Can you work these out from the model? Positions are in its coordinate system, mm. Face numbers are marked on the shaded views. A direction names the side the tool comes from. Give positions to 0.01 mm unless a question says otherwise; leave off trailing zeros. Loops run counter-clockwise (first coordinate to the right, second up) from the corner with the lowest first, then second, coordinate; pieces in that order, holes last. Notation, with made-up numbers: (36.25, 16.25) - (94.25, 16.25) arc R36 cw to (94.25, 51.25) - close; hole circle Ø10 at (16.25, 34). An arc over 180 degrees is marked (long way). Write item = value, one per line.
from build123d import *

# Parameters (mm, degrees)
RESSALTO_EXTRUS_O1_DEPTH      = 0.8
RESSALTO_EXTRUS_O2_DEPTH      = 1
RESSALTO_EXTRUS_O2_DEPTH_BACK = 6


with BuildPart() as part:
    # Esboço1 → Ressalto-extrusão1 (new body)
    with BuildSketch(Plane.XY):
        Polygon((8.5, 13.5), (-8.5, 13.5), (-8.5, -13.5), (-6.5, -13.5), (-6.5, -11.5), (6.5, -11.5), (6.5, -13.5), (8.5, -13.5), align=None)
    extrude(amount=RESSALTO_EXTRUS_O1_DEPTH)

    # Esboço3 → Ressalto-extrusão2 (add, two sides)
    with BuildSketch(Plane(origin=(0, 13.5, 0), x_dir=(1, 0, 0), z_dir=(0, 1, 0))) as ressalto_extrus_o2_sk:
        with BuildLine():
            Line((-3, 3), (3, 3))
            ThreePointArc((3, 3), (4.5, 1.5), (3, 0))
            Line((3, 0), (-3, 0))
            ThreePointArc((-3, 0), (-4.5, 1.5), (-3, 3))
        make_face()
    extrude(amount=RESSALTO_EXTRUS_O2_DEPTH)
    extrude(ressalto_extrus_o2_sk.sketch, amount=-RESSALTO_EXTRUS_O2_DEPTH_BACK)


solid = part.part
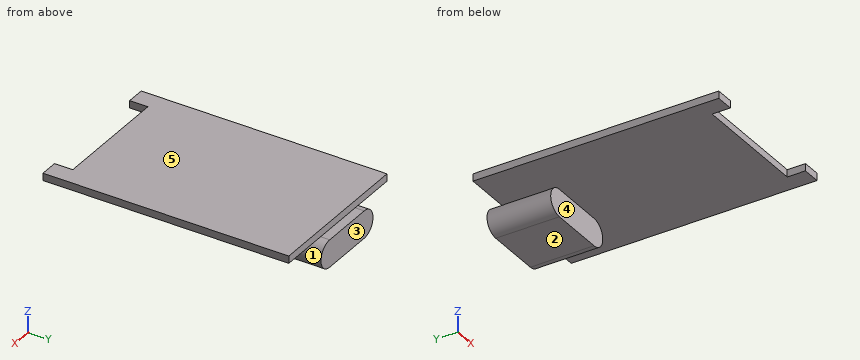
Q1. For pin 1 (8.5 mm diameter, centred on x = -1.5, y = -4.5, fed in from -Z); pin 2 (0.9 mm diameter, centred on x = 1.5, z = -1, fed in from -Y); pin 3 (0.8 mm diameter, centred on x = 1, y = 14, fed in from +Z), each with a flat end and sliding along its axis, tell me the tip position at first contact or that it passes through.
Output:
pin_1 = 0
pin_2 = 7.5
pin_3 = 0
Q2. Imagine slicing it at B-B, the plane y = -3.5. Write out the boundary of the cut face in (x, z), then the cut area to 3 significant figures.
Output:
outline = (-8.5, 0) - (8.5, 0) - (8.5, 0.8) - (-8.5, 0.8) - close
area = 13.6 mm2
Q3. Imagine slicing it at A-A, the plane z = 0.5. Write out the boundary of the cut face in (x, y), then the cut area to 3 significant figures.
Output:
outline = (-8.5, -13.5) - (-6.5, -13.5) - (-6.5, -11.5) - (6.5, -11.5) - (6.5, -13.5) - (8.5, -13.5) - (8.5, 13.5) - (-8.5, 13.5) - close
area = 433 mm2
Q4. We'd pull the mould along Z, two halves only. Please class the marked faces 1, 2 and 3: released by +Z, released by -Z, zero draft, split by the parting line, or undercut.
Output:
face_1 = undercut
face_2 = released by -Z
face_3 = zero draft
Q5. I need wall thicknesses on L1, parallel to Z at x = 6.25, y = -10.75; L2, parallel to Y at x = -2.25, z = -0.05; L3, parallel to Y at x = 0.25, z = 0.2. Which ranges of each line are inside material? Lowest first, please.
Output:
L1 = 0 to 0.8
L2 = 7.5 to 14.5
L3 = -11.5 to 13.5
Q6. Which directions (+Z, -Z, +X, -X, +Y, -Y) give clear straight access to the entire face, cutting with the end or side of a thin tool? Please do the marked faces 4 and 5.
Output:
face_4 = -Z, +X, -X, -Y
face_5 = +Z, +X, -X, +Y, -Y
Q7. Imagine slicing it at C-C, the plane x = 6. Write out the boundary of the cut face in (y, z).
Output:
outline = (-11.5, 0) - (13.5, 0) - (13.5, 0.8) - (-11.5, 0.8) - close
